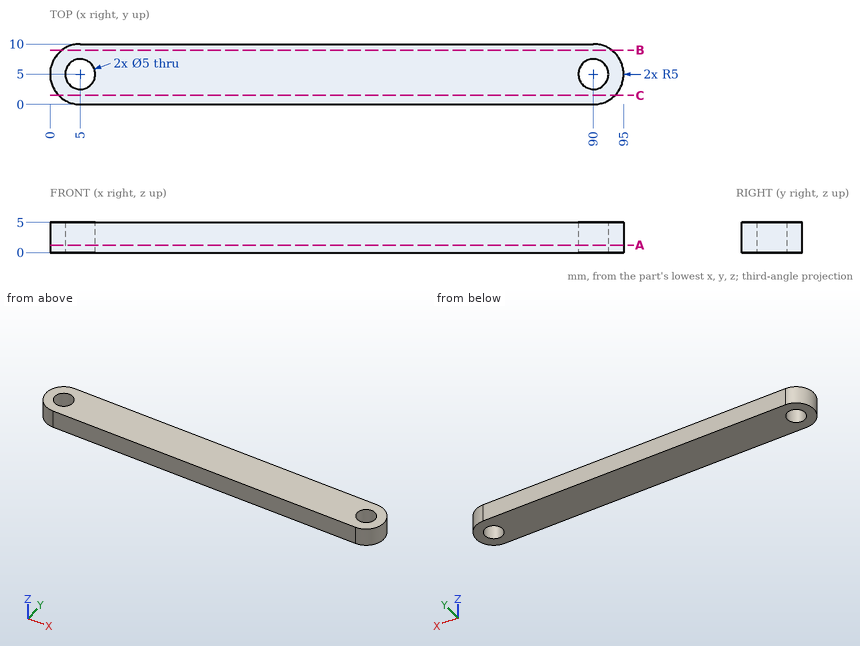
Input: dimensioned drawing with shaded views. Units: mm. Origin: part minimum x, y, z. Coordinates: 2 decimals unless noted, no trailing zeros. Loops run counter-clockwise (first coordinate to the right, second up) from the corner with the lowest first, then second, coordinate; pieces in that order, holes last.
Q1. Section C-C, the plane y = 1.5. Return the cut outline in (x, z), and give its area (3 significant figures).
Results are:
outline: (1.43, 0) - (93.57, 0) - (93.57, 5) - (1.43, 5) - close
area: 461 mm2
Q2. Section B-B, the plane y = 9. Return the cut outline in (x, z).
Results are:
outline: (2, 0) - (93, 0) - (93, 5) - (2, 5) - close
Q3. Contact query for flat-ended pins moving along their axis: pin 1 (5 mm diameter, centred on x = 58.5, y = 2, fed in from -Z); pin 2 (3 mm diameter, centred on y = 2, z = 1.5, fed in from +X). Output: stop coordinate, or through.
Results are:
pin 1: stops at z = 0
pin 2: stops at x = 94.77
Q4. Line query: line 1 along Y through (x, z) = (5, 2.25); line 2 along X through (y, z) = (3.25, 2.8); line 3 along X through (y, z) = (4.5, 1.55). Output: solid intervals per line, ascending.
Results are:
line 1: y = 0 to 2.5, 7.5 to 10
line 2: x = 0.32 to 3.21, 6.79 to 88.21, 91.79 to 94.68
line 3: x = 0.03 to 2.55, 7.45 to 87.55, 92.45 to 94.97
Q5. Section A-A, the plane z = 1.25. Return the cut outline in (x, y).
Results are:
outline: (5, 0) - (90, 0) arc R5 ccw to (90, 10) - (5, 10) arc R5 ccw to start; hole circle Ø5 at (5, 5); hole circle Ø5 at (90, 5)
